Here's how the part is built. I have some questions about the finished solid (model axes, mm). A direction names the side the tool comes from. Give positions to 0.01 mm unless a question says otherwise; leave off trailing zeros. Write each loop counter-clockwise with the first axis right and the second up, starting at its lowest first coordinate (ties: lowest second). Pieces come first, ordered by that corner, then holes. Notation, with made-up numbers: (44, 36) - (66, 36) arc R20 cw to (66, 50) - close; hole circle Ø1 at (29.5, 13). An arc over 180 degrees is marked (long way). Use a Markdown table: item, result.
```python
from build123d import *

# Parameters (mm, degrees)
SKETCH2_W             = 33.02
SKETCH2_H             = 33.02
BOSS_EXTRUDE2_DEPTH   = 5.334
SKETCH3_W             = 33.02
SKETCH3_H             = 5.334
BOSS_EXTRUDE6_DEPTH   = 5.334
SKETCH6_W             = 11.006666666
SKETCH6_H             = 5.334
CUT_EXTRUDE2_DEPTH    = 32.349198203
CAVITY2_START         = -21.844
CAVITY2_OUTLINE_W     = 5.334
CAVITY2_OUTLINE_H     = 13.208
CAVITY2_OUTLINE_H_2   = 12.573
CAVITY2_DEPTH         = 5.334
CAVITY2_START_2       = 16.51
CAVITY2_2_OUTLINE_W   = 5.334
CAVITY2_2_OUTLINE_H   = 13.208
CAVITY2_2_OUTLINE_H_2 = 12.573
CAVITY2_2_DEPTH       = 5.334
CAVITY2_START_3       = -7.281333333
CAVITY2_3_OUTLINE_W   = 5.334
CAVITY2_3_OUTLINE_H   = 5.334
CAVITY2_3_DEPTH       = 14.562666666
SKETCH7_R             = 1.5
SKETCH7_R_2           = 4.953
CUT_EXTRUDE3_DEPTH    = 32.349198203


# Read off the part's stored shape, not the designer's step: Cavity2
with BuildPart() as part:
    # Sketch2 → Boss-Extrude2 (new body)
    with BuildSketch(Plane(origin=(0, 0, 0), x_dir=(0, 0, -1), z_dir=(1, 0, 0))):
        Rectangle(SKETCH2_W, SKETCH2_H)
    extrude(amount=BOSS_EXTRUDE2_DEPTH)

    # Sketch3 → Boss-Extrude6 (add, through all)
    with BuildSketch(Plane(origin=(5.334, 0, 0), x_dir=(0, 0, -1), z_dir=(1, 0, 0))):
        Polygon((-16.51, 16.51), (-16.51, 21.844), (-21.844, 21.844), (-21.844, -16.51), (-16.51, -16.51), align=None)
        with Locations((0, 19.177)):
            Rectangle(SKETCH3_W, SKETCH3_H)
        Polygon((21.844, 21.844), (21.844, -16.51), (16.51, -16.51), (16.51, 16.51), (16.51, 21.844), align=None)
        with Locations((0, -19.177)):
            Rectangle(SKETCH3_W, SKETCH3_H)
    extrude(amount=-BOSS_EXTRUDE6_DEPTH)

    # Sketch6 → Cut-Extrude2 (cut, through all)
    with BuildSketch(Plane(origin=(5.334, 0, 0), x_dir=(0, 0, -1), z_dir=(1, 0, 0))):
        with Locations((0, -19.177)):
            Rectangle(SKETCH6_W, SKETCH6_H)
    extrude(amount=-CUT_EXTRUDE2_DEPTH, mode=Mode.SUBTRACT)

    # Cavity2 outline → Cavity2 (cut)
    with BuildSketch(Plane.XY.offset(CAVITY2_START)):
        with Locations((2.667, -9.906)):
            Rectangle(CAVITY2_OUTLINE_W, CAVITY2_OUTLINE_H)
        with Locations((2.667, 15.5575)):
            Rectangle(CAVITY2_OUTLINE_W, CAVITY2_OUTLINE_H_2)
    extrude(amount=CAVITY2_DEPTH, mode=Mode.SUBTRACT)

    # Cavity2 2 outline → Cavity2 2 (cut)
    with BuildSketch(Plane.XY.offset(CAVITY2_START_2)):
        with Locations((2.667, -9.906)):
            Rectangle(CAVITY2_2_OUTLINE_W, CAVITY2_2_OUTLINE_H)
        with Locations((2.667, 15.5575)):
            Rectangle(CAVITY2_2_OUTLINE_W, CAVITY2_2_OUTLINE_H_2)
    extrude(amount=CAVITY2_2_DEPTH, mode=Mode.SUBTRACT)

    # Cavity2 3 outline → Cavity2 3 (cut)
    with BuildSketch(Plane.XY.offset(CAVITY2_START_3)):
        with Locations((2.667, 19.177)):
            Rectangle(CAVITY2_3_OUTLINE_W, CAVITY2_3_OUTLINE_H)
    extrude(amount=CAVITY2_3_DEPTH, mode=Mode.SUBTRACT)

    # Sketch7 → Cut-Extrude3 (cut, through all)
    with BuildSketch(Plane.ZY):
        with Locations((0, 13.51)):
            Circle(SKETCH7_R)
        with Locations((11.75, -6.841596989)):
            Circle(SKETCH7_R)
        with Locations((0, -6.604)):
            Circle(SKETCH7_R_2)
        with Locations((-11.75, -6.841596989)):
            Circle(SKETCH7_R)
    extrude(amount=-CUT_EXTRUDE3_DEPTH, mode=Mode.SUBTRACT)


solid = part.part
```
Item 1: If we section it at B-B, the plane y = -17.5: Write out the boundary of the cut face in (x, z).
Values:
| item | result |
|---|---|
| outline | (0, -16.51) - (5.33, -16.51) - (5.33, -5.5) - (0, -5.5) - close; (0, 5.5) - (5.33, 5.5) - (5.33, 16.51) - (0, 16.51) - close |
Item 2: Thinking about a two-plate mould opening in Z: for faces 6 (the flat face through (3, 3, -21.844)), 7 (the flat face through (3, -19, -5.503)), 8 (the cylindrical face through (2.63, 12.046, -0.325)), 9 (the flat face through (3, -3.302, -19)), which applies, +Z half, -Z half, draft (parallel to the pull), parting line (faces both ways), or undercut?
Values:
| item | result |
|---|---|
| face 6 | -Z half |
| face 7 | undercut |
| face 8 | undercut |
| face 9 | draft |
Item 3: If we section it at D-D, the plane x = 1.5: Write out the boundary of the cut face in (y, z), plus the area to 3 significant figures.
Values:
| item | result |
|---|---|
| outline | (-21.84, -16.51) - (-3.3, -16.51) - (-3.3, -21.84) - (9.27, -21.84) - (9.27, -16.51) - (21.84, -16.51) - (21.84, -7.28) - (16.51, -7.28) - (16.51, 7.28) - (21.84, 7.28) - (21.84, 16.51) - (9.27, 16.51) - (9.27, 21.84) - (-3.3, 21.84) - (-3.3, 16.51) - (-21.84, 16.51) - (-21.84, 5.5) - (-16.51, 5.5) - (-16.51, -5.5) - (-21.84, -5.5) - close; hole circle Ø9.91 at (-6.6, 0); hole circle Ø3 at (-6.84, -11.75); hole circle Ø3 at (-6.84, 11.75); hole circle Ø3 at (13.51, 0) |
| area | 1,340 mm2 |
Item 4: If we section it at C-C, the plane z = -11.75: Write out the boundary of the cut face in (x, y), plus the area to 3 significant figures.
Values:
| item | result |
|---|---|
| outline | (0, -21.84) - (5.33, -21.84) - (5.33, -8.34) - (0, -8.34) - close; (0, -5.34) - (5.33, -5.34) - (5.33, 21.84) - (0, 21.84) - close |
| area | 217 mm2 |
Item 5: I need wall thicknesses on line 1 along Y through (x, z) = (3.2, 0); line 2 along Y through (x, z) = (3.2, -11.75); line 3 along Z through (x, y) = (4, -17.5). Which ranges of each line are inside material? Lowest first, please. Write a range as [from, to].
Values:
| item | result |
|---|---|
| line 1 | y = [-16.51, -11.56], [-1.65, 12.01], [15.01, 16.51] |
| line 2 | y = [-21.84, -8.34], [-5.34, 21.84] |
| line 3 | z = [-16.51, -5.5], [5.5, 16.51] |
Item 6: If we section it at A-A, the plane z = 0: Write out the boundary of the cut face in (x, y).
Values:
| item | result |
|---|---|
| outline | (0, -16.51) - (5.33, -16.51) - (5.33, -11.56) - (0, -11.56) - close; (0, -1.65) - (5.33, -1.65) - (5.33, 12.01) - (0, 12.01) - close; (0, 15.01) - (5.33, 15.01) - (5.33, 16.51) - (0, 16.51) - close |
Item 7: Will these pins go through, and if not, where does the flat tip stop? pin 1 Ø5 at (y, z) = (-6.84, -11.75) entering from -X; pin 2 Ø1.6 at (x, y) = (1.5, -18) entering from +Z; pin 3 Ø1.5 at (x, z) = (2, 2) entering from -Y; pin 4 Ø2.5 at (x, z) = (1.5, -20.5) entering from -Y.
Values:
| item | result |
|---|---|
| pin 1 | stops at x = 0 |
| pin 2 | stops at z = 16.51 |
| pin 3 | stops at y = -16.51 |
| pin 4 | stops at y = -3.3 |
Item 8: For faces 1 (the flat face through (3, 9.271, 19)), 2 (the flat face through (3, -3.302, 19)), 3 (the flat face through (3, -16.51, 0)), 4 (the flat face through (3, 19, 7.281)), 5 (the flat face through (3, 9.271, -19)), which set-ups out of +Z, -Z, +X, -X, +Y, -Y let a thin tool reach every point of the face, with its end or its side?
Values:
| item | result |
|---|---|
| face 1 | +Z, +X, -X, +Y |
| face 2 | +Z, +X, -X, -Y |
| face 3 | +X, -X, -Y |
| face 4 | +X, -X, +Y |
| face 5 | -Z, +X, -X, +Y |
